The listing builds one solid part. Answer for the finished solid, in the listing's coordinates (mm). Face numbers are marked on the shaded views. Coordinates: 2 decimals unless noted, no trailing zeros. Loops run counter-clockwise (first coordinate to the right, second up) from the corner with the lowest first, then second, coordinate; pieces in that order, holes last. Notation, with made-up numbers: (11, -14.75) - (32, -14.75) arc R22 ccw to (32, -0.75) - close; hole circle Ø11 at (-22, -12.75). An arc over 180 degrees is marked (long way). Return JSON: item names as keys, results as strings. Group by question number.
1. Section B-B (y = 4.15) is taken. Write down the section's boundary in (x, z), and give its area (3 significant figures).
2. Section D-D (x = -10) is taken. Write down the section's boundary in (y, z), and give its area (3 significant figures).
3. Section C-C (x = 0) is taken. Write down the section's boundary in (y, z).
4. The mould has two halves that part along X. Classify the marked faces 1 and 2: pulls with the +X half, pulls with the -X half, needs draft (parallel to the pull), parting line crosses it, or undercut.
5. Each of these flat-tipped pins is pushed along its axis until it touches: P1, Ø0.8, axis at x = -41.5, y = 3, coming from the -Z side (3 decimals); P2, Ø10, axis at x = -26, z = 2, coming from the +Y side; P3, Ø1.3, axis at y = 5, z = -19, coming from the +X side. Where does it stop, or does it pass through?
6. Section A-A (z = -12) is taken. Write down the section's boundary in (x, y).
7. Find the intervals of material crossed by line 1 along X through (y, z) = (1.5, -7.5); line 2 along X through (y, z) = (1.2, 9); line 3 along Z through (x, y) = (9, 0.9), in increasing order.
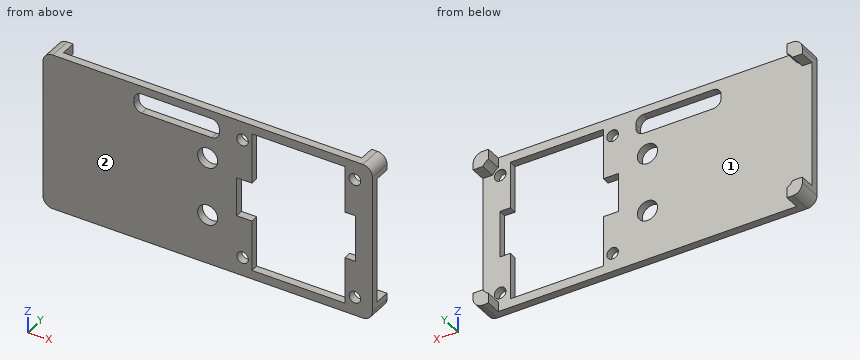
Autodesk Inventor part; units mm, degrees
ref_plane "YZ Plane" through (0, 0, 0) normal (1, 0, 0) x (0, 1, 0)
ref_plane "XZ Plane" through (0, 0, 0) normal (0, 1, 0) x (-1, 0, 0)
ref_plane "XY Plane" through (0, 0, 0) normal (0, 0, 1) x (1, 0, 0)
sketch "草图3" plane through (0, 0, 0) normal (0, 1, 0) x (-1, 0, 0)
  line L0 (40, 20.25) -> (-40, 20.25)
  line L1 (-42.5, 17.75) -> (-42.5, -17.75)
  line L2 (-40, -20.25) -> (40, -20.25)
  line L3 (42.5, -17.75) -> (42.5, 17.75)
  line L4 (42.5, 20.25) -> (-42.5, -20.25) construction
  line L5 (-42.5, 20.25) -> (42.5, -20.25) construction
  arc A0 (42.5, 17.75) -> (40, 20.25) centre (40, 17.75) ccw
  arc A1 (-40, 20.25) -> (-42.5, 17.75) centre (-40, 17.75) ccw
  arc A2 (-42.5, -17.75) -> (-40, -20.25) centre (-40, -17.75) ccw
  arc A3 (40, -20.25) -> (42.5, -17.75) centre (40, -17.75) ccw
  circle A4 centre (40.5, 18.25) radius 1
  line L6 (42.5, 0) -> (50.0267, 0)
  circle A5 centre (40.5, -18.25) radius 1
  line L7 (0, 0) -> (0, 15.1914)
  circle A6 centre (-40.5, 18.25) radius 1
  circle A7 centre (-40.5, -18.25) radius 1
  line L8 (42.5, 20.25) -> (38.5, 20.25)
  line L9 (38.5, 20.25) -> (38.5, 16.25)
  line L10 (38.5, 16.25) -> (42.5, 16.25)
  line L11 (42.5, 16.25) -> (42.5, 20.25)
  line L12 (42.5, 20.25) -> (38.5, 16.25) construction
  line L13 (38.5, 20.25) -> (42.5, 16.25) construction
  line L14 (42.5, -16.25) -> (38.5, -16.25)
  line L15 (38.5, -16.25) -> (38.5, -20.25)
  line L16 (38.5, -20.25) -> (42.5, -20.25)
  line L17 (42.5, -20.25) -> (42.5, -16.25)
  line L18 (42.5, -16.25) -> (38.5, -20.25) construction
  line L19 (38.5, -16.25) -> (42.5, -20.25) construction
  line L20 (-38.5, 20.25) -> (-42.5, 20.25)
  line L21 (-42.5, 20.25) -> (-42.5, 16.25)
  line L22 (-42.5, 16.25) -> (-38.5, 16.25)
  line L23 (-38.5, 16.25) -> (-38.5, 20.25)
  line L24 (-38.5, 20.25) -> (-42.5, 16.25) construction
  line L25 (-42.5, 20.25) -> (-38.5, 16.25) construction
  line L26 (-38.5, -16.25) -> (-42.5, -16.25)
  line L27 (-42.5, -16.25) -> (-42.5, -20.25)
  line L28 (-42.5, -20.25) -> (-38.5, -20.25)
  line L29 (-38.5, -20.25) -> (-38.5, -16.25)
  line L30 (-38.5, -16.25) -> (-42.5, -20.25) construction
  line L31 (-42.5, -16.25) -> (-38.5, -20.25) construction
  line L32 (-36.5, 18.25) -> (36.5, 18.25)
  arc A8 (40.5, 17.75) -> (40, 18.25) centre (40, 17.75) ccw
  line L33 (40.5, 14.25) -> (40.5, -14.25)
  arc A9 (40, -18.25) -> (40.5, -17.75) centre (40, -17.75) ccw
  line L34 (36.5, -18.25) -> (-36.5, -18.25)
  arc A10 (-40.5, -17.75) -> (-40, -18.25) centre (-40, -17.75) ccw
  line L35 (-40.5, -14.25) -> (-40.5, 14.25)
  arc A11 (-40, 18.25) -> (-40.5, 17.75) centre (-40, 17.75) ccw
  arc A12 (-40.5, -14.25) -> (-36.5, -18.25) centre (-36.5, -14.25) ccw
  arc A13 (-36.5, 18.25) -> (-40.5, 14.25) centre (-36.5, 14.25) ccw
  arc A14 (40.5, 14.25) -> (36.5, 18.25) centre (36.5, 14.25) ccw
  arc A15 (36.5, -18.25) -> (40.5, -14.25) centre (36.5, -14.25) ccw
  point P0 (-38.5, -17.7141)
  point P1 (-39.9641, -16.25)
  point P2 (-39.9641, 16.25)
  point P3 (-38.5, 17.7141)
  point P4 (39.9641, -16.25)
  point P5 (38.5, -17.7141)
  point P6 (38.5, 17.7141)
  point P7 (39.9641, 16.25)
  dimension "d11" = 85
  dimension "d12" = 40.5
  dimension "d13" = 2.5
  dimension "d14" = 2
  dimension "d15" = 2
  dimension "d16" = 2
  dimension "d72" = 4
  dimension "d73" = 4
  dimension "d74" = 4
  dimension "d75" = 4
  dimension "d76" = 4
  dimension "d77" = 4
  dimension "d78" = 4
  dimension "d79" = 4
  dimension "d80" = 2
  dimension "d81" = 4
extrude "拉伸3" add sketch "草图3" along normal blind 2 contours A0 L3 L10 A14 L9 L0 | L9 A14 L32 A13 L23 L0 | L23 A13 L22 L1 A1 L0 | A14 L10 L9 | L9 L10 A14 L33 A15 L14 L15 L34 A12 L29 L26 L35 A13 L22 L23 L32 | L3 L14 A15 L33 A14 L10 | L23 L22 A13 | A13 L35 A12 L26 L1 L22 | L3 A3 L2 L15 A15 L14 | A15 L15 L14 | L26 A12 L29 L2 A2 L1 | L15 L2 L29 A12 L34 A15 | L26 L29 A12 | A4 | A5 | A6 | A7
extrude "拉伸4" add sketch "草图3" along normal blind 6 contours A0 L3 L10 A14 L9 L0 | L8 L11 A0 | L23 A13 L22 L1 A1 L0 | A1 L21 L20 | L3 A3 L2 L15 A15 L14 | L17 L16 A3 | L26 A12 L29 L2 A2 L1 | A2 L28 L27 | A4 | A5 | A6 | A7
sketch "草图4" plane through (0, 0, 0) normal (0, -1, 0) x (1, 0, 0)
  line L0 (40.5, -20.1774) -> (40.5, 20.25)
  line L1 (-38.5, 20.25) -> (38.5, 20.25)
  line L2 (42.5, 17.75) -> (42.5, -17.75)
  line L3 (38.5, -20.25) -> (-38.5, -20.25)
  line L4 (6.5, -20.25) -> (6.5, 20.25)
  circle A0 centre (38, -15.5) radius 1.5
  line L5 (40.5, -18) -> (25.2781, -18)
  line L6 (25.2781, -18) -> (6.5, -18)
  line L7 (6.5, 18) -> (40.5, 18)
  line L8 (23.5, 18) -> (23.5, -18)
  circle A1 centre (9, -15.5) radius 1.5
  circle A2 centre (9, 15.5) radius 1.5
  circle A3 centre (38, 15.5) radius 1.5
  line L9 (11.4, -18) -> (11.4, 18)
  line L10 (35.4, -18) -> (35.4, 18)
  line L11 (35.4, -6) -> (38.1, -6)
  line L12 (38.1, -6) -> (38.1, 6)
  line L13 (38.1, 6) -> (35.4, 6)
  line L14 (6.5, -5) -> (9.5, -5)
  line L15 (9.5, -5) -> (9.5, 5)
  line L16 (9.5, 5) -> (6.5, 5)
  line L17 (7.5, -5) -> (11.5, -5)
  line L18 (11.5, -5) -> (11.5, 5)
  line L19 (11.5, 5) -> (7.5, 5)
  line L20 (7.5, 5) -> (7.5, -5)
  line L21 (7.5, -5) -> (11.5, 5) construction
  line L22 (11.5, -5) -> (7.5, 5) construction
  point P0 (0, 0)
  point P1 (-40, 20.25)
  point P2 (40, 20.25)
  point P3 (40, -20.25)
  point P4 (-40, -20.25)
  point P5 (9.5, 0)
  point P6 (7.5, 5)
  point P7 (7.5, -5)
  dimension "d21" = 2
  dimension "d22" = 34
  dimension "d23" = 3
  dimension "d24" = 2.5
  dimension "d25" = 18
  dimension "d26" = 2.5
  dimension "d27" = 18
  dimension "d28" = 3
  dimension "d29" = 3
  dimension "d30" = 3
  dimension "d31" = 2.5
  dimension "d32" = 2.5
  dimension "d33" = 2.5
  dimension "d34" = 2.5
  dimension "d35" = 2.5
  dimension "d36" = 2.5
  dimension "d37" = 2.4
  dimension "d38" = 24
  dimension "d39" = 2.7
  dimension "d40" = 6
  dimension "d41" = 12
  dimension "d42" = 3
  dimension "d43" = 5
  dimension "d44" = 10
  dimension "d45" = 4
  dimension "d46" = 10
extrude "拉伸5" cut sketch "草图4" against normal blind 2 contours L5 L6 L8 L7 L10 | L10 L13 L12 L11 | L8 L6 L9 L17 L18 L19 L7 | L19 L18 L17 L9 | L9 L17 L15 L19 | L15 L14 L20 L16 | A0 | A1 | A2 | A3
fillet "圆角6" radius 2.5 4 edges at (-42.5, 3, -20.25) (-42.5, 3, 20.25) (42.5, 3, 20.25) (42.5, 3, -20.25)
sketch "草图6" plane through (0, 0, 0) normal (0, -1, 0) x (1, 0, 0)
  line L0 (-40, 20.25) -> (40, 20.25)
  line L1 (0, 20.25) -> (-19, 20.25)
  line L2 (-19, 20.25) -> (-19, 13.25)
  line L3 (-19, 13.25) -> (0, 13.25)
  line L4 (0, 13.25) -> (0, 20.25)
  line L5 (0, 13.25) -> (3, 13.25)
  line L6 (3, 13.25) -> (3, 20.25)
  line L7 (3, 20.25) -> (0, 20.25)
  line L8 (0, 20.25) -> (0, 13.25)
  line L9 (3, 20.25) -> (3, 18.25)
  line L10 (3, 18.25) -> (-19, 18.25)
  point P0 (0, 0)
  dimension "d83" = 19
  dimension "d84" = 7
  dimension "d85" = 3
  dimension "d86" = 7
  dimension "d87" = 2
extrude "拉伸7" cut sketch "草图6" against normal blind 2 contours L10 L4 L3 L2 | L10 L6 L5 L4
fillet "圆角7" radius 2 4 edges at (3, 1, 13.25) (3, 1, 18.25) (-19, 1, 13.25) (-19, 1, 18.25)
sketch "草图7" plane through (0, 0, 0) normal (0, -1, 0) x (1, 0, 0)
  circle A0 centre (0, 0) radius 7.5
  circle A1 centre (0, -7.5) radius 2.6
  circle A2 centre (0, 7.5) radius 2.6
  dimension "d91" = 5.2
  dimension "d92" = 5.2
extrude "拉伸8" cut sketch "草图7" against normal blind 2 contours A2 A0 | A0 A2 | A1 A0 | A0 A1
properties part number "盖" material "聚碳酸酯，透明"
The answers:
{
 "1": {"outline": "(-42.5, -17.75) arc R2.5 ccw to (-40, -20.25) - (-38.5, -20.25) - (-38.5, -17.71) arc R4 cw to (-39.96, -16.25) - (-42.5, -16.25) - close; (-42.5, 16.25) - (-39.96, 16.25) arc R4 cw to (-38.5, 17.71) - (-38.5, 20.25) - (-40, 20.25) arc R2.5 ccw to (-42.5, 17.75) - close; (38.5, -20.25) - (40, -20.25) arc R2.5 ccw to (42.5, -17.75) - (42.5, -16.25) - (39.96, -16.25) arc R4 cw to (38.5, -17.71) - close; (38.5, 17.71) arc R4 cw to (39.96, 16.25) - (42.5, 16.25) - (42.5, 17.75) arc R2.5 ccw to (40, 20.25) - (38.5, 20.25) - close", "area": "53.6 mm2"},
 "2": {"outline": "(0, -20.25) - (2, -20.25) - (2, 13.25) - (0, 13.25) - close; (0, 18.25) - (2, 18.25) - (2, 20.25) - (0, 20.25) - close", "area": "71.0 mm2"},
 "3": {"outline": "(0, -20.25) - (2, -20.25) - (2, -10.1) - (0, -10.1) - close; (0, -4.9) - (2, -4.9) - (2, 4.9) - (0, 4.9) - close; (0, 10.1) - (2, 10.1) - (2, 13.25) - (0, 13.25) - close; (0, 18.25) - (2, 18.25) - (2, 20.25) - (0, 20.25) - close"},
 "4": {"face 1": "undercut", "face 2": "needs draft"},
 "5": {"P1": "stops at z = -19.995", "P2": "stops at y = 2", "P3": "stops at x = 42.43"},
 "6": {"outline": "(-42.5, 0) - (11.4, 0) - (11.4, 2) - (-42.5, 2) - close; (35.4, 0) - (42.5, 0) - (42.5, 2) - (35.4, 2) - close"},
 "7": {"line 1": "x = -42.5 to -2.6, 2.6 to 11.4, 35.4 to 42.5", "line 2": "x = -42.5 to -2.12, 2.12 to 11.4, 35.4 to 42.5", "line 3": "z = -20.25 to -17, -14 to -5, 5 to 14, 17 to 20.25"}
}
